from build123d import *

# Parameters (mm, degrees)
SKETCH1_W           = 2438.4
SKETCH1_H           = 88.9
BOSS_EXTRUDE1_DEPTH = 38.1
CUT_EXTRUDE1_DEPTH  = 89.9
SKETCH3_W           = 84.1375
SKETCH3_H           = 50.8
CUT_EXTRUDE2_DEPTH  = 39.1


with BuildPart() as part:
    # Sketch1 → Boss-Extrude1 (new body)
    with BuildSketch(Plane(origin=(0, 0, 0), x_dir=(1, 0, 0), z_dir=(0, 1, 0))):
        with Locations((1219.2, 44.45)):
            Rectangle(SKETCH1_W, SKETCH1_H)
    extrude(amount=BOSS_EXTRUDE1_DEPTH)

    # Sketch2 → Cut-Extrude1 (cut, through all)
    with BuildSketch(Plane.XY):
        Polygon((0, 0), (38.1, 38.1), (0, 38.1), align=None)
        Polygon((2438.4, 0), (2438.4, 38.1), (2400.3, 38.1), align=None)
    extrude(amount=-CUT_EXTRUDE1_DEPTH, mode=Mode.SUBTRACT)

    # Sketch3 → Cut-Extrude2 (cut, through all)
    with BuildSketch(Plane(origin=(0, 38.1, 0), x_dir=(1, 0, 0), z_dir=(0, 1, 0))):
        with Locations((1920.08125, 25.4)):
            Rectangle(SKETCH3_W, SKETCH3_H)
    extrude(amount=-CUT_EXTRUDE2_DEPTH, mode=Mode.SUBTRACT)


solid = part.part
Build history of the part. All positions in model axes, mm. A direction names the side the tool comes from. Coordinates: 2 decimals unless noted, no trailing zeros. Write each loop counter-clockwise with the first axis right and the second up, starting at its lowest first coordinate (ties: lowest second). Pieces come first, ordered by that corner, then holes.
(1) Cut at A-A on z = -30. List the corners of the cut face in (x, y), and give its area (3 significant figures).
(2) Pin check, flat tips, straight feed: pin 1 Ø3 at (y, z) = (28, -39) entering from -X; pin 2 Ø5 at (y, z) = (10.5, -32) entering from -X; pin 3 Ø10 at (y, z) = (23.5, -51.5) entering from +X; pin 4 Ø3 at (x, y) = (1389, 23.5) entering from +Z. Stop position of each tip, or through.
(3) Cut at B-B on y = 19. List the corners of the cut face in (x, z).
(4) Mould opens along X. For faces 3 (the flat face through (19, 19, -44)), 4 (the flat face through (1919, 19, -50.8)), 5 (the flat face through (1202, 0, -45)) say: pulls with the +X half, pulls with the -X half, needs draft (parallel to the pull), parting line crosses it, or undercut.
(5) 3-axis set-ups, long thin cutter, end or side, ignore diameter. For faces 1 (the flat face through (1962.15, 19, -25)), 2 (the flat face through (926, 19, 0)): which of +Z, -Z, +X, -X, +Y, -Y reach the whole face in a straight line?
(6) Drill centre lines: line 1 (X direction, y = 34.5, z = -12.5); line 2 (X direction, y = 10.5, z = -26); line 3 (X direction, y = 14.5, z = -80.5). Where is each one in solid material? Low to high.
Working result:
1. outline: (0, 0) - (1878.01, 0) - (1878.01, 38.1) - (38.1, 38.1) - close; (1962.15, 0) - (2438.4, 0) - (2400.3, 38.1) - (1962.15, 38.1) - close
1. area: 88,200 mm2
2. pin 1: stops at x = 26.5
2. pin 2: stops at x = 8
2. pin 3: stops at x = 2419.9
2. pin 4: stops at z = 0
3. outline: (19, -88.9) - (2419.4, -88.9) - (2419.4, 0) - (1962.15, 0) - (1962.15, -50.8) - (1878.01, -50.8) - (1878.01, 0) - (19, 0) - close
4. face 3: pulls with the -X half
4. face 4: undercut
4. face 5: needs draft
5. face 1: +Z, +Y, -Y
5. face 2: +Z, +X, -X, +Y, -Y
6. line 1: x = 34.5 to 1878.01, 1962.15 to 2403.9
6. line 2: x = 10.5 to 1878.01, 1962.15 to 2427.9
6. line 3: x = 14.5 to 2423.9
